Check sheet for the modelled part. Datum: model origin and axes. Units: mm. Round coordinates to 2 decimals unless told otherwise and drop trailing zeros. Loops run counter-clockwise (first coordinate to the right, second up) from the corner with the lowest first, then second, coordinate; pieces in that order, holes last. Notation, with made-up numbers: M 22,49.25 L 34,49.25 A22 cw 34,76.25 Z; hole C 84.25,0.5 d8. An arc over 180 degrees is marked long. Write item = value, one per line. Start each with the question number.
(1) Cross-section at B-B on x = 297. Record the boundary of the cut face in (y, z), plus the area to 3 significant figures.
(2) Scan lines: L1, parallel to Y at x = 360, z = 2.1; L2, parallel to X at y = 74, z = 2.75; L3, parallel to X at y = 12, z = 2.6. Record each from-to range of solid material in increasing order. Write a range as from..to.
(3) Cross-section at D-D on x = 245.5. Record the boundary of the cut face in (y, z).
(4) Cross-section at C-C on z = 1.65. State how many separate pieces and enclosed holes the cut face has, plus the area to 3 significant figures.
(5) Go/stop test with flat-tipped pins: P1, Ø1.5, axis at x = 366, z = 1, coming from the -Y side; P2, Ø1.2, axis at x = 362.5, z = 1, coming from the -Y side; P3, Ø0.9, axis at y = 92.5, z = 1.5, coming from the +X side. Record where each tip stops, or that it passes through.
(6) Cross-section at A-A on y = 74.5. Record the boundary of the cut face in (x, z).
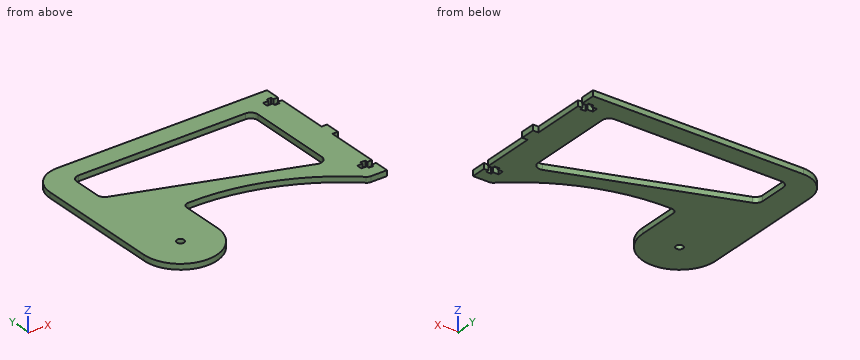
from build123d import *

# Parameters (mm, degrees)
SKETCH_1_R      = 2
EXTRUDE_1_DEPTH = 3


with BuildPart() as part:
    # 草图1 → 凸台-拉伸1 (new body)
    with BuildSketch(Plane.XY):
        with BuildLine():
            Line((364.002581869, 97.707860978), (354.002581869, 97.707860978))
            Line((354.002581869, 97.707860978), (249.002581869, 97.707860978))
            ThreePointArc((249.002581869, 97.707860978), (238.395980151, 93.314462696), (234.002581869, 82.707860978))
            Line((234.002581869, 82.707860978), (234.002581869, 13.707860978))
            ThreePointArc((234.002581869, 13.707860978), (254.002581869, -6.292139022), (274.002581869, 13.707860978))
            Line((274.002581869, 13.707860978), (274.002581869, 35.819123465))
            ThreePointArc((274.002581869, 35.819123465), (274.855620398, 37.914488932), (276.929619495, 38.818236083))
            ThreePointArc((276.929619495, 38.818236083), (317.768023154, 31.985283132), (353.154233351, 10.484571811))
            ThreePointArc((353.154233351, 10.484571811), (354.089046944, 9.908765811), (355.16842929, 9.707860978))
            Line((355.16842929, 9.707860978), (364.002581869, 9.707860978))
            Line((364.002581869, 9.707860978), (364.002581869, 17.707860978))
            Line((364.002581869, 17.707860978), (361.502581869, 17.707860978))
            Line((361.502581869, 17.707860978), (361.502581869, 16.207860978))
            Line((361.502581869, 16.207860978), (358.902581869, 16.207860978))
            Line((358.902581869, 16.207860978), (358.902581869, 17.707860978))
            Line((358.902581869, 17.707860978), (355.902581869, 17.707860978))
            Line((355.902581869, 17.707860978), (355.902581869, 20.707860978))
            Line((355.902581869, 20.707860978), (358.902581869, 20.707860978))
            Line((358.902581869, 20.707860978), (358.902581869, 22.207860978))
            Line((358.902581869, 22.207860978), (361.502581869, 22.207860978))
            Line((361.502581869, 22.207860978), (361.502581869, 20.707860978))
            Line((361.502581869, 20.707860978), (364.002581869, 20.707860978))
            Line((364.002581869, 20.707860978), (364.002581869, 49.707860978))
            Line((364.002581869, 49.707860978), (367.002581869, 49.707860978))
            Line((367.002581869, 49.707860978), (367.002581869, 57.707860978))
            Line((367.002581869, 57.707860978), (364.002581869, 57.707860978))
            Line((364.002581869, 57.707860978), (364.002581869, 86.707860978))
            Line((364.002581869, 86.707860978), (361.502581869, 86.707860978))
            Line((361.502581869, 86.707860978), (361.502581869, 85.207860978))
            Line((361.502581869, 85.207860978), (358.902581869, 85.207860978))
            Line((358.902581869, 85.207860978), (358.902581869, 86.707860978))
            Line((358.902581869, 86.707860978), (355.902581869, 86.707860978))
            Line((355.902581869, 86.707860978), (355.902581869, 89.707860978))
            Line((355.902581869, 89.707860978), (358.902581869, 89.707860978))
            Line((358.902581869, 89.707860978), (358.902581869, 91.207860978))
            Line((358.902581869, 91.207860978), (361.502581869, 91.207860978))
            Line((361.502581869, 91.207860978), (361.502581869, 89.707860978))
            Line((361.502581869, 89.707860978), (364.002581869, 89.707860978))
            Line((364.002581869, 89.707860978), (364.002581869, 97.707860978))
        make_face()
        with Locations((254.002581869, 13.707860978)):
            Circle(SKETCH_1_R, mode=Mode.SUBTRACT)
        with BuildLine():
            Line((253.002581869, 86.967009497), (344.129272471, 86.967009497))
            ThreePointArc((344.129272471, 86.967009497), (346.957699596, 85.795436622), (348.129272471, 82.967009497))
            Line((348.129272471, 82.967009497), (348.129272471, 36.172406577))
            ThreePointArc((348.129272471, 36.172406577), (346.444858552, 32.910802508), (342.810241921, 32.396144085))
            Line((342.810241921, 32.396144085), (251.683551319, 64.226264226))
            ThreePointArc((251.683551319, 64.226264226), (249.740977801, 65.686940637), (249.002581869, 68.002526718))
            Line((249.002581869, 68.002526718), (249.002581869, 82.967009497))
            ThreePointArc((249.002581869, 82.967009497), (250.174154745, 85.795436622), (253.002581869, 86.967009497))
        make_face(mode=Mode.SUBTRACT)
    extrude(amount=EXTRUDE_1_DEPTH)


solid = part.part
Result:
q1.outline = M 37.46,0 L 48.4,0 L 48.4,3 L 37.46,3 Z; M 86.97,0 L 97.71,0 L 97.71,3 L 86.97,3 Z
q1.area = 65.0 mm^2
q2.L1 = 9.71..16.21, 22.21..85.21, 91.21..97.71
q2.L2 = 234..249, 348.13..364
q2.L3 = 234.08..252.96, 255.04..273.93, 351.45..364
q3.outline = M -4.39,0 L 97.29,0 L 97.29,3 L -4.39,3 Z
q4.separate_pieces = 1
q4.enclosed_holes = 2
q4.area = 6,300 mm^2
q5.P1 = 49.71
q5.P2 = 9.71
q5.P3 = 364
q6.outline = M 234,0 L 249,0 L 249,3 L 234,3 Z; M 348.13,0 L 364,0 L 364,3 L 348.13,3 Z
